Solid Edge part; units mm, degrees
sketch "Sketch1" plane through (0, 0, 0) normal (0, -1, 0) x (1, 0, 0)
  circle A0 centre (0, 0) radius 4
  circle A1 centre (0, 0) radius 6
extrude "Protrusion1" add sketch "Sketch1" against normal blind 7
sketch "Sketch2" plane through (0, 0, 0) normal (0, 0, 1) x (1, 0, 0)
  circle A0 centre (7.75, 3.5) radius 2
revolve "RevolvedCutout1" cut sketch "Sketch2" angle 360 about axis through (0, 0, 0) along (0, 1, 0)
chamfer "Chanfrein_1" distance 0.25 angle 45 2 edges at (-6, 7, 0) (-6, 0, 0)
chamfer "Chanfrein_2" distance 0.5 angle 45 2 edges at (-4, 0, 0) (-4, 7, 0)
properties material "Steel"
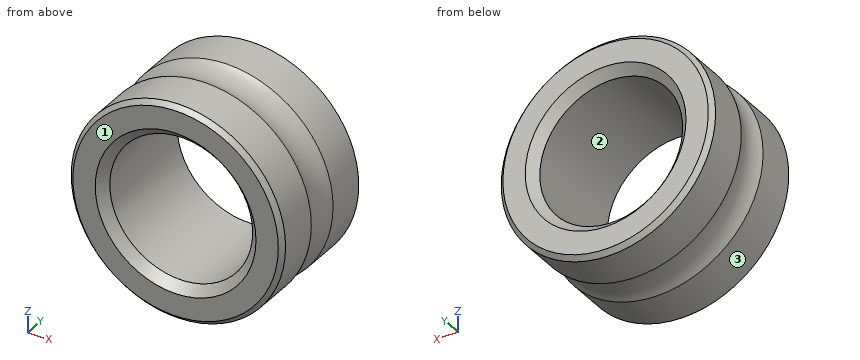
Model file for the job. Use its own axes, mm. Face numbers are marked on the shaded views. Give positions to 0.01 mm unless a question says otherwise; leave off trailing zeros. Order: outer loops, then holes, each group sorted by start corner. A loop starts at its lowest first (then second) coordinate and runs counter-clockwise, first axis right, second up.
1) Pin check, flat tips, straight feed: pin 1 (2 mm diameter, centred on y = 1, z = 4.5, fed in from -X); pin 2 (1 mm diameter, centred on y = 3, z = -2, fed in from +X); pin 3 (4 mm diameter, centred on y = 5.5, z = -4, fed in from -X). Stop position of each tip, or through.
2) Saw through at A-A, the plane x = 0. Write the cut outline in (y, z), then the cut area to 3 significant figures.
3) Saw through at C-C, the plane y = 1. Write the cut outline in (x, z), then the cut area to 3 significant figures.
4) Wall check: probe 1 along Z at (x, y) = (0, 3.55); probe 2 along Z at (x, y) = (0, 1.7); probe 3 along X at (y, z) = (4.5, 1). Give the ranges that are in metal, low to high.
5) Mould opens along X. For the marked faces 1, 2 and 3 say: +X half, -X half, draft (parallel to the pull), parting line (faces both ways), or undercut.
6) Saw through at B-B, the plane z = 0. Write the cut outline in (x, y), then the cut area to 3 significant figures.
7) Saw through at D-D, the plane y = 4. Write the cut outline in (x, z), then the cut area to 3 significant figures.
Computed:
1. pin 1: stops at x = -4.87
1. pin 2: stops at x = 5.72
1. pin 3: stops at x = -5.66
2. outline: (0, -5.75) - (0.25, -6) - (2.53, -6) arc R2 cw to (4.47, -6) - (6.75, -6) - (7, -5.75) - (7, -4.5) - (6.5, -4) - (0.5, -4) - (0, -4.5) - close; (0, 4.5) - (0.5, 4) - (6.5, 4) - (7, 4.5) - (7, 5.75) - (6.75, 6) - (4.47, 6) arc R2 cw to (2.53, 6) - (0.25, 6) - (0, 5.75) - close
2. area: 26.7 mm2
3. outline: circle Ø12 at (0, 0); hole circle Ø8 at (0, 0)
3. area: 62.8 mm2
4. probe 1: z = -5.75 to -4, 4 to 5.75
4. probe 2: z = -6 to -4, 4 to 6
4. probe 3: x = -5.92 to -3.87, 3.87 to 5.92
5. face 1: draft
5. face 2: undercut
5. face 3: parting line
6. outline: (-6, 0.25) - (-5.75, 0) - (-4.5, 0) - (-4, 0.5) - (-4, 6.5) - (-4.5, 7) - (-5.75, 7) - (-6, 6.75) - (-6, 4.47) arc R2 cw to (-6, 2.53) - close; (4, 0.5) - (4.5, 0) - (5.75, 0) - (6, 0.25) - (6, 2.53) arc R2 cw to (6, 4.47) - (6, 6.75) - (5.75, 7) - (4.5, 7) - (4, 6.5) - close
6. area: 26.7 mm2
7. outline: circle Ø11.63 at (0, 0); hole circle Ø8 at (0, 0)
7. area: 55.9 mm2
